Answer from the drawing. Dimensions are ordinates in mm from the lowest x, y and z of the part. A direction names the side the tool comes from. Coordinates: 2 decimals unless noted, no trailing zeros. Write each loop counter-clockwise with the first axis right and the second up, starting at its lowest first coordinate (ties: lowest second). Pieces come first, ordered by that corner, then holes.
(1) Section D-D on z = 20.75 is taken. Write down the section's boundary in (x, y), then the cut area to 3 significant figures.
(2) Which of the six approach directions +Z, -Z, +X, -X, +Y, -Y give full straight-line access (tool end or side, diameter ignored) to the marked faces 4, 5 and 6?
(3) Section C-C on x = 28 is taken. Write down the section's boundary in (y, z) (3 decimals), then the cut area to 3 significant figures.
(4) Find the intervals of material crossed by probe 1 along Z at (x, y) = (44, 106) (3 decimals); probe 2 along X at (y, z) = (124.5, 10); probe 3 along Z at (x, y) = (14, 61.5) (3 decimals), in increasing order.
(5) The mould has two halves that part along X. Classify the marked faces 1, 2 and 3: +X half, -X half, draft (parallel to the pull), parting line (faces both ways), or undercut.
(6) Given pin 1 (6.5 mm diameter, centred on x = 23, z = 13, fed in from -Y); pin 2 (10.5 mm diameter, centred on x = 63, y = 40, fed in from -Z) (3 decimals); pin 3 (2 mm diameter, centred on x = 57.5, z = 14, fed in from +Y); pin 4 (8 mm diameter, centred on y = 22.5, z = 13, fed in from -X), each flat-ended and moving along its own axis, determine where each tip first touches the part or whether it passes through.
(7) Section A-A on x = 44.45 is taken. Write down the section's boundary in (y, z) (3 decimals).
(8) Section B-B on z = 13.25 is taken. Write down the section's boundary in (x, y), then the cut area to 3 significant figures.
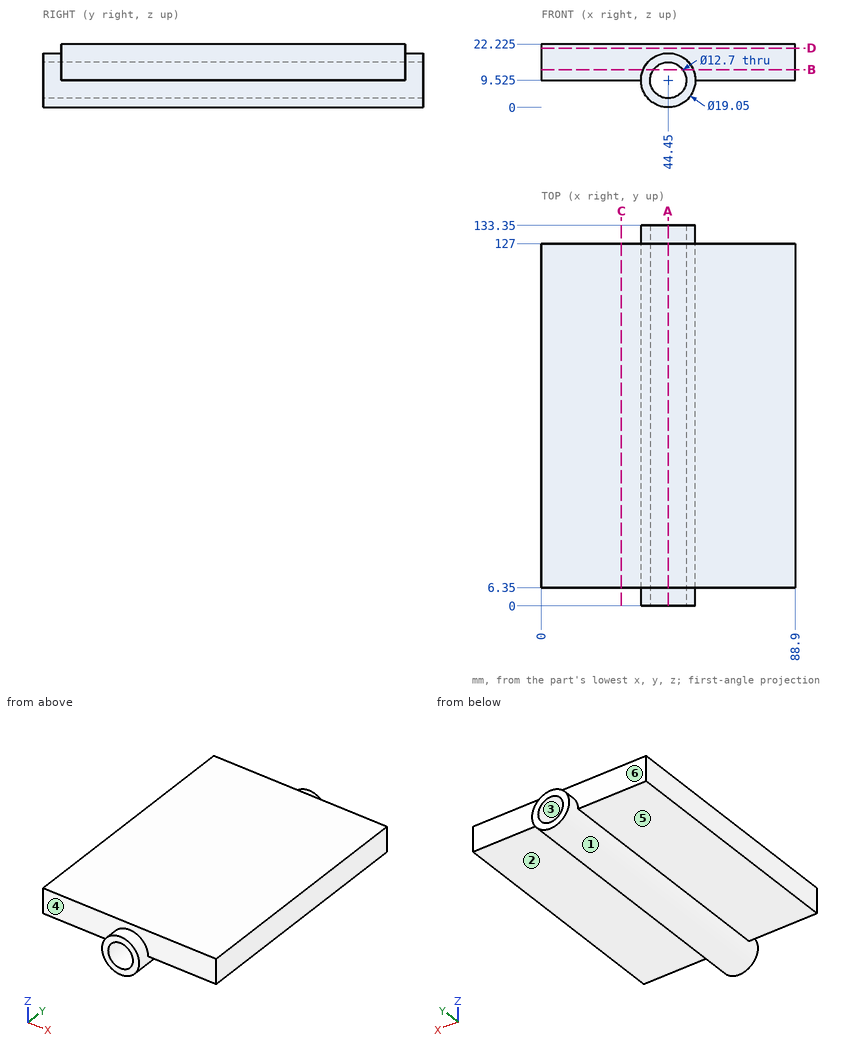
Response:
1. outline: (0, 6.35) - (88.9, 6.35) - (88.9, 127) - (0, 127) - close
1. area: 10,700 mm2
2. face 4: +Z, -Y
2. face 5: -Z, -X, +Y, -Y
2. face 6: +Z, +Y
3. outline: (6.35, 9.525) - (127, 9.525) - (127, 22.225) - (6.35, 22.225) - close
3. area: 1,530 mm2
4. probe 1: z = 0.011 to 3.191, 15.859 to 22.225
4. probe 2: x = 0 to 38.12, 50.78 to 88.9
4. probe 3: z = 9.525 to 22.225
5. face 1: parting line
5. face 2: draft
5. face 3: undercut
6. pin 1: stops at y = 6.35
6. pin 2: stops at z = 9.525
6. pin 3: stops at y = 127
6. pin 4: stops at x = 0
7. outline: (0, 0) - (133.35, 0) - (133.35, 3.175) - (0, 3.175) - close; (0, 15.875) - (133.35, 15.875) - (133.35, 19.05) - (127, 19.05) - (127, 22.225) - (6.35, 22.225) - (6.35, 19.05) - (0, 19.05) - close
8. outline: (0, 6.35) - (35.68, 6.35) - (35.68, 0) - (39.31, 0) - (39.31, 133.35) - (35.68, 133.35) - (35.68, 127) - (0, 127) - close; (49.59, 0) - (53.22, 0) - (53.22, 6.35) - (88.9, 6.35) - (88.9, 127) - (53.22, 127) - (53.22, 133.35) - (49.59, 133.35) - close
8. area: 9,580 mm2
